Geometry: final body of the model. Coordinates: model frame, mm. Coordinates: 2 decimals unless noted, no trailing zeros. Loops run counter-clockwise (first coordinate to the right, second up) from the corner with the lowest first, then second, coordinate; pieces in that order, holes last. Notation, with made-up numbers: (70.25, -12.5) - (124.25, -12.5) arc R25 cw to (124.25, 0.5) - close; hole circle Ø2 at (-7.5, -31.5). An arc over 180 degrees is marked (long way). Return JSON: item names as keys, results as strings.
from build123d import *

# Parameters (mm, degrees)
F1_DEPTH = 4
F2_W     = 47.4
F2_H     = 4
F2_W_2   = 4
F2_H_2   = 21
F2_H_3   = 25
F3_DEPTH = 4
F5_DEPTH = 4


with BuildPart() as f1:
    # F0 (on Front) → F1 (new body)
    with BuildSketch(Plane.XZ):
        with BuildLine():
            Line((0, 150), (0, 0))
            Line((0, 0), (237, 0))
            Line((237, 0), (237, 150))
            ThreePointArc((237, 150), (222.355339, 185.355339), (187, 200))
            Line((187, 200), (50, 200))
            ThreePointArc((50, 200), (14.644661, 185.355339), (0, 150))
        make_face()
    extrude(amount=F1_DEPTH)

    # F2 (on face) → F3 (cut, through all)
    with BuildSketch(Plane.XZ.offset(4)):
        Polygon((0, 4), (0, 0), (47.4, 0), (47.4, 4), (4, 4), align=None)
        Polygon((189.6, 4), (189.6, 0), (237, 0), (237, 4), (233, 4), align=None)
        with Locations((118.5, 2)):
            Rectangle(F2_W, F2_H)
        with Locations((2, 14.5)):
            Rectangle(F2_W_2, F2_H_2)
        with Locations((235, 14.5)):
            Rectangle(F2_W_2, F2_H_2)
        with Locations((2, 87.5)):
            Rectangle(F2_W_2, F2_H_3)
        with Locations((235, 87.5)):
            Rectangle(F2_W_2, F2_H_3)
    extrude(amount=-F3_DEPTH, mode=Mode.SUBTRACT)

    # F4 (on face) → F5 (cut, through all)
    with BuildSketch(Plane.XZ.offset(4)):
        with BuildLine():
            Line((183.5, 180), (53.5, 180))
            ThreePointArc((53.5, 180), (46.428932, 177.071068), (43.5, 170))
            Line((43.5, 170), (43.5, 160))
            ThreePointArc((43.5, 160), (46.428932, 152.928932), (53.5, 150))
            Line((53.5, 150), (183.5, 150))
            ThreePointArc((183.5, 150), (190.571068, 152.928932), (193.5, 160))
            Line((193.5, 160), (193.5, 170))
            ThreePointArc((193.5, 170), (190.571068, 177.071068), (183.5, 180))
        make_face()
    extrude(amount=-F5_DEPTH, mode=Mode.SUBTRACT)


solid = f1.part
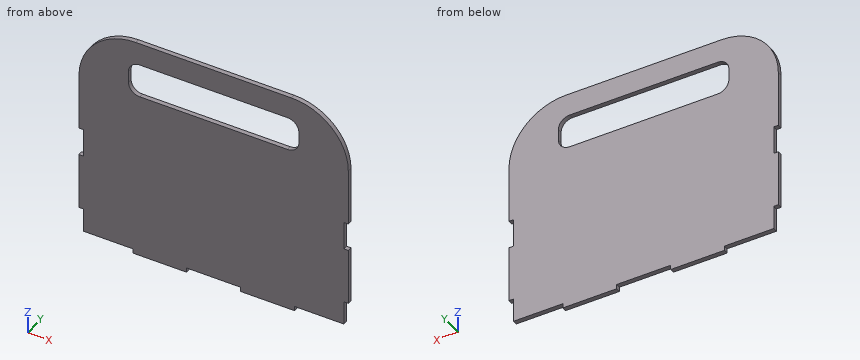
Item 1: Ray query, probe 1 along Z at (x, y) = (101.5, -3.4); probe 2 along Z at (x, y) = (156, -2.8); probe 3 along Z at (x, y) = (10, -0.8). Return the intervals inside material, ascending. Write a range as from..to.
Worked out:
{"probe 1": "4..150, 180..200", "probe 2": "0..150, 180..200", "probe 3": "4..180"}
Item 2: Section query C-C, the plane x = 200. Return loops of the section in (y, z), and give its area (3 significant figures).
Worked out:
{"outline": "(-4, 4) - (0, 4) - (0, 198.28) - (-4, 198.28) - close", "area": "777 mm^2"}
Item 3: First-contact query: pin 1 Ø2 at (x, y) = (27, -1) entering from +Z; pin 2 Ø2 at (x, y) = (220, -1) entering from -Z; pin 3 Ø2 at (y, z) = (-1.5, 2.5) entering from +X. Flat tips, straight axial feed; report the tip coordinate or a pass-through.
Worked out:
{"pin 1": "z = 194.9", "pin 2": "z = 4", "pin 3": "x = 189.6"}
Item 4: Section query A-A, the plane x = 98. Return loops of the section in (y, z), and give its area (3 significant figures).
Worked out:
{"outline": "(-4, 4) - (0, 4) - (0, 150) - (-4, 150) - close; (-4, 180) - (0, 180) - (0, 200) - (-4, 200) - close", "area": "664 mm^2"}
